Autodesk Inventor part; units mm, degrees
ref_plane "YZ Plane" through (0, 0, 0) normal (1, 0, 0) x (0, 1, 0)
ref_plane "XZ Plane" through (0, 0, 0) normal (0, 1, 0) x (-1, 0, 0)
ref_plane "XY Plane" through (0, 0, 0) normal (0, 0, 1) x (1, 0, 0)
sketch "Sketch1" plane through (0, 0, 0) normal (0, 0, 1) x (1, 0, 0)
  line L0 (0, 0) -> (6, 0)
  line L1 (6, 0) -> (6, 11)
  line L2 (0, 0) -> (0, 15)
  line L3 (0, 15) -> (2, 15)
  line L4 (2, 15) -> (6, 11)
  dimension "d0" = 6
  dimension "d1" = 11
  dimension "d2" = 15
  dimension "d3" = 2
extrude "Extrusion1" add sketch "Sketch1" along normal blind 10
sketch "Sketch2" plane through (0, 0, 10) normal (0, 0, 1) x (1, 0, 0)
  line L0 (0, 15) -> (0, 0)
  line L1 (0, 0) -> (6, 0)
  line L2 (6, 11) -> (2, 15)
  line L3 (0, 11) -> (3, 8)
  line L4 (0, 11) -> (-3, 8)
  line L5 (-3, 8) -> (-3, 0)
  line L6 (2, 15) -> (0, 15)
  line L7 (0, 15) -> (2, 15)
  line L8 (6, 0) -> (6, 11)
  line L9 (2, 15) -> (6, 11)
  line L10 (6, 11) -> (6, 0)
  line L11 (6, 0) -> (0, 0)
  line L12 (0, 0) -> (-6, 0)
  line L13 (-6, 11) -> (-2, 15)
  line L14 (-2, 15) -> (0, 15)
  line L15 (-6, 0) -> (-6, 11)
  line L16 (3, 8) -> (3, 0)
  line L17 (3, 0) -> (6, 0)
  line L18 (-3, 0) -> (-6, 0)
  line L19 (0, 11) -> (0, 15)
  dimension "d6" = 3
extrude "Extrusion2" add sketch "Sketch2" along normal blind 26 contours L6 L2 L8 L1 L16 L3 L0 | L0 L4 L5 L12 L15 L13 L14
sketch "Sketch3" plane through (0, 0, 36) normal (0, 0, 1) x (1, 0, 0)
  line L0 (2, 15) -> (-2, 15)
  line L1 (0, 15) -> (2, 15)
  line L2 (6, 11) -> (2, 15)
  line L3 (2, 15) -> (6, 11)
  line L4 (6, 0) -> (6, 11)
  line L5 (6, 11) -> (6, 0)
  line L6 (0, 0) -> (6, 0)
  line L7 (6, 0) -> (0, 0)
  line L8 (0, 15) -> (0, 11)
  line L9 (0, 0) -> (0, 15)
extrude "Extrusion3" add sketch "Sketch3" along normal blind 10
properties part number "outside-join"
Check sheet for the modelled part. Datum: model origin and axes. Units: mm. A direction names the side the tool comes from. Give positions to 0.01 mm unless a question says otherwise; leave off trailing zeros. Write each loop counter-clockwise with the first axis right and the second up, starting at its lowest first coordinate (ties: lowest second). Pieces come first, ordered by that corner, then holes.
Item 1: Cross-section at C-C (z = 25). Enter the section's corners in (x, y).
Item 2: Cross-section at B-B (x = 0.5). Enter the section's corners in (y, z), and give its area (3 significant figures).
Item 3: Cross-section at D-D (y = 11.5). Enter the section's corners in (x, z), and give its area (3 significant figures).
Item 4: Scan lines: L1, parallel to X at y = 7.5, z = 13; L2, parallel to Z at x = 2.25, y = 5; L3, parallel to X at y = 4.25, z = 6.5. Record each from-to range of solid material in increasing order.
Item 5: Draft check along Z on faces 1 (the face through (-4, 13, 23)), 2 (the face through (3, 8, 46)), 3 (the face through (3, 4, 23)), 4 (the face through (1, 4, 10)). Enter one of: released by +Z, released by -Z, zero draft, split by the parting line, or undercut.
Item 6: Gauge pin test, flat ends, axial feed: pin 1 (8 mm diameter, centred on y = 9, z = 41.5, fed in from -X); pin 2 (4 mm diameter, centred on x = -3, y = 13, fed in from -Z). Record the tip position at first contact, or that the pin passes through.
Item 7: Access from +Z, -Z, +X, -X, +Y, -Y to the whole of each face (thin tool, end or side, straight path). Record for faces 5 (the face through (0, 7, 5)), 6 (the face through (-3, 4, 23)), 7 (the face through (1, 4, 36)).
Item 8: Cross-section at A-A (y = 8.75). Enter the section's corners in (x, z).
Report:
1. outline: (-6, 0) - (-3, 0) - (-3, 8) - (0, 11) - (3, 8) - (3, 0) - (6, 0) - (6, 11) - (2, 15) - (-2, 15) - (-6, 11) - close
2. outline: (0, 0) - (15, 0) - (15, 46) - (0, 46) - (0, 36) - (10.5, 36) - (10.5, 10) - (0, 10) - close
2. area: 417 mm2
3. outline: (-5.5, 10) - (0, 10) - (0, 0) - (5.5, 0) - (5.5, 46) - (0, 46) - (0, 36) - (-5.5, 36) - close
3. area: 396 mm2
4. L1: x = -6 to -3, 3 to 6
4. L2: z = 0 to 10, 36 to 46
4. L3: x = 0 to 6
5. face 1: zero draft
5. face 2: released by +Z
5. face 3: undercut
5. face 4: undercut
6. pin 1: stops at x = 0
6. pin 2: stops at z = 10
7. face 5: -Z, -X, +Y, -Y
7. face 6: +Z, -Z, -Y
7. face 7: -Y
8. outline: (-6, 10) - (-2.25, 10) - (-2.25, 36) - (-6, 36) - close; (0, 0) - (6, 0) - (6, 46) - (0, 46) - (0, 36) - (2.25, 36) - (2.25, 10) - (0, 10) - close
